Could you check a few things on this model? Use its own coordinates, in mm. Face numbers are marked on the shaded views. A direction names the side the tool comes from. Coordinates: 2 decimals unless noted, no trailing zeros. Order: outer loops, then holes, each group sorted by start corner. A loop starts at its lowest first (then second) coordinate and runs counter-clockwise, first axis right, second up. Notation, with made-up numbers: (21, -32.75) - (45, -32.75) arc R16 cw to (45, -24.75) - close; hole circle Ø7 at (-34, 74). An arc over 180 degrees is marked (long way). One line per item, written item: value.
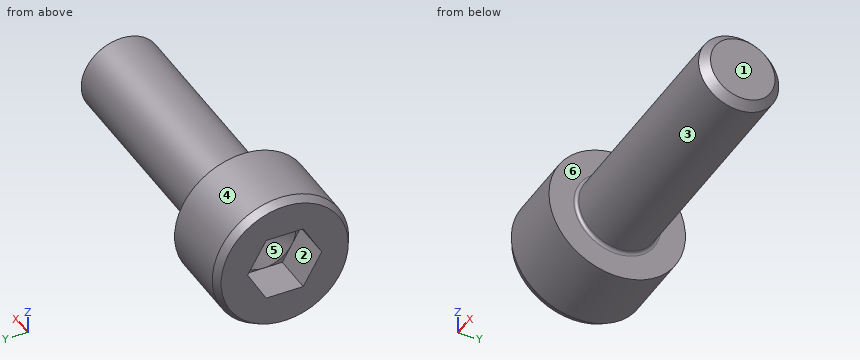
from build123d import *

# Parameters (mm, degrees)
CUT_EXTRUDE_1_DEPTH = 2.5


with BuildPart() as part:
    # Sketch 1 → Revolve 1 (revolve)
    with BuildSketch(Plane.XY, mode=Mode.PRIVATE) as revolve_1_sk:
        with BuildLine():
            Line((-5, 0), (-5, 3.961324865))
            Line((-5, 3.961324865), (-4.5, 4.25))
            Line((-4.5, 4.25), (0, 4.25))
            Line((0, 4.25), (0, 2.7))
            ThreePointArc((0, 2.7), (0.058578644, 2.558578644), (0.2, 2.5))
            Line((0.2, 2.5), (14.5095, 2.5))
            Line((14.5095, 2.5), (15, 2.0095))
            Line((15, 2.0095), (15, 0))
            Line((15, 0), (-5, 0))
        make_face()
    revolve(revolve_1_sk.sketch.rotate(Axis((15, 0, 0), (-1, 0, 0)), 180), axis=Axis((15, 0, 0), (-1, 0, 0)))

    # Sketch 2 → Cut-Revolve 1 (revolve, cut)
    with BuildSketch(Plane.XY, mode=Mode.PRIVATE) as cut_revolve_1_sk:
        Polygon((-5, 0), (-5, 2), (-2.5, 2), (-1.345299462, 0), align=None)
    revolve(cut_revolve_1_sk.sketch.rotate(Axis((-1.345299462, 0, 0), (-1, 0, 0)), 270), axis=Axis((-1.345299462, 0, 0), (-1, 0, 0)), mode=Mode.SUBTRACT)

    # Sketch 3 → Cut-Extrude 1 (cut)
    with BuildSketch(Plane(origin=(-5, 0, 0), x_dir=(0, 0, -1), z_dir=(1, 0, 0))):
        Polygon((-2, -1.154700538), (0, -2.309401077), (2, -1.154700538), (2, 1.154700538), (0, 2.309401077), (-2, 1.154700538), align=None)
    extrude(amount=CUT_EXTRUDE_1_DEPTH, mode=Mode.SUBTRACT)


solid = part.part
Item 1: If I drill on probe 1 along Y at (x, z) = (2.75, -1.5); probe 2 along Z at (x, y) = (3.5, 0); probe 3 along X at (y, z) = (-3.5, -0.5), over which ranges is the centre line in solid material (lowest first)?
Conclusion:
probe 1: -2 to 2
probe 2: -2.5 to 2.5
probe 3: -5 to 0
Item 2: Thinking about a two-plate mould opening in Y: for the marked faces 4, 5 and 6, which applies, pulls with the +Y half, pulls with the -Y half, needs draft (parallel to the pull), parting line crosses it, or undercut?
Conclusion:
face 4: parting line crosses it
face 5: undercut
face 6: needs draft
Item 3: I'm going to push flat-ended pins straight in: pin 1 Ø0.7 at (x, y) = (-3.5, 0.5) entering from -Z; pin 2 Ø5 at (x, y) = (12, 1) entering from -Z; pin 3 Ø4 at (x, z) = (10, 1.5) entering from +Y. Where does each tip first touch, or does it pass through?
Conclusion:
pin 1: z = -4.25
pin 2: z = -2.5
pin 3: y = 2.5
Item 4: For the marked faces 1, 2 and 3, which set-ups out of +Z, -Z, +X, -X, +Y, -Y let a thin tool reach every point of the face, with its end or its side?
Conclusion:
face 1: +Z, -Z, +X, +Y, -Y
face 2: -X
face 3: +X
Item 5: I want a section at A-A on x = 7.25. Please give me the cut outline in (y, z).
Conclusion:
outline: circle Ø5 at (0, 0)
